Build history of the part. All positions in model axes, mm. Face numbers are marked on the shaded views. A direction names the side the tool comes from. Round coordinates to 2 decimals unless told otherwise and drop trailing zeros. Write each loop counter-clockwise with the first axis right and the second up, starting at its lowest first coordinate (ties: lowest second). Pieces come first, ordered by that corner, then holes. Notation, with made-up numbers: M -22.75,-38 L -14.75,-38 A28 ccw -14.75,-4 Z; hole C -24.75,28.25 d2. An arc over 180 degrees is marked long. Write item = value, one per line.
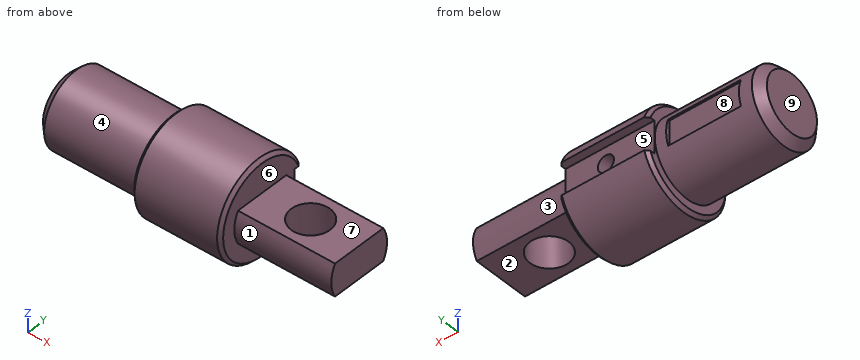
from build123d import *

# Parameters (mm, degrees)
SKETCH_2_W                  = 45
SKETCH_2_H                  = 2.5
CUT_EXTRUDE_1_DEPTH         = 8
SKETCH_4_W                  = 20
SKETCH_4_H                  = 6.715728753
CUT_EXTRUDE_2_DEPTH         = 123.576506721
HOLE_WIZARD_10_0_10_1_D     = 10
HOLE_WIZARD_10_0_10_1_DEPTH = 35
HOLE_WIZARD_10_0_10_1_TIP   = 3.004303095
CUT_EXTRUDE_START           = -60
CUT_EXTRUDE_3_DEPTH         = 245.932420089
HOLE_WIZARD_24_0_24_1_D     = 24
CHAMFER_1_SIZE              = 5
CHAMFER_2_SIZE              = 2


with BuildPart() as part:
    # Эскиз1 → Повернуть1 (revolve)
    with BuildSketch(Plane.XY, mode=Mode.PRIVATE) as revolve_1_sk:
        Polygon((0, 0), (0, 23), (65, 23), (65, 30), (120, 30), (120, 20), (180, 20), (180, 0), align=None)
    revolve(revolve_1_sk.sketch.rotate(Axis((0, 0, 0), (-1, 0, 0)), 90), axis=Axis((0, 0, 0), (-1, 0, 0)))

    # Эскиз2 → Вырез-Вытянуть1 (cut, symmetric)
    with BuildSketch(Plane.XY):
        with Locations((35.5, 21.75)):
            Rectangle(SKETCH_2_W, SKETCH_2_H)
    extrude(amount=CUT_EXTRUDE_1_DEPTH, both=True, mode=Mode.SUBTRACT)

    # Эскиз4 → Вырез-Вытянуть2 (cut, through all)
    with BuildSketch(Plane.ZY.offset(-65)):
        with Locations((0, 26.642135624)):
            Rectangle(SKETCH_4_W, SKETCH_4_H)
    extrude(amount=-CUT_EXTRUDE_2_DEPTH, mode=Mode.SUBTRACT)

    # Диаметр отверстия Ø10.0 (10)1
    with Locations(Plane(origin=(0, 23.284271247, 0), x_dir=(1, 0, 0), z_dir=(0, 1, 0))):
        with Locations((95, 0)):
            Hole(HOLE_WIZARD_10_0_10_1_D / 2, depth=HOLE_WIZARD_10_0_10_1_DEPTH)
            with Locations((0, 0, -(HOLE_WIZARD_10_0_10_1_DEPTH + HOLE_WIZARD_10_0_10_1_TIP / 2))):  # 118° drill point
                Cone(0, HOLE_WIZARD_10_0_10_1_D / 2, HOLE_WIZARD_10_0_10_1_TIP, mode=Mode.SUBTRACT)

    # Эскиз7 → Вырез-Вытянуть3 (cut)
    with BuildSketch(Plane(origin=(180, 0, 0), x_dir=(0, 0, -1), z_dir=(1, 0, 0)).offset(CUT_EXTRUDE_START)):
        Polygon((-10, 151.24355653), (-10, 17.320508076), (-10, -17.320508076), (-10, -151.24355653), (-277.846096908, -151.24355653), (-277.846096908, 151.24355653), align=None)
    cut_extrude_3 = extrude(amount=CUT_EXTRUDE_3_DEPTH, mode=Mode.SUBTRACT)

    # Зеркальное отражение1: Вырез-Вытянуть3 across plane
    add(cut_extrude_3.mirror(Plane.XY), mode=Mode.SUBTRACT)

    # Диаметр отверстия Ø24.0 (24)1 (through all)
    with Locations(Plane.XY.offset(10)):
        with Locations((150, 0)):
            Hole(HOLE_WIZARD_24_0_24_1_D / 2)

    # Фаска1
    chamfer_1_edges = [part.edges().sort_by_distance(p)[0] for p in [
        (0, 0, 23),
    ]]
    chamfer(chamfer_1_edges, length=CHAMFER_1_SIZE)

    # Фаска2
    chamfer_2_edges = [part.edges().sort_by_distance(p)[0] for p in [
        (120, -30, 0),
        (65, -30, 0),
    ]]
    chamfer(chamfer_2_edges, length=CHAMFER_2_SIZE)


solid = part.part
1. Band-saw the part on C-C (x = 63). List the corners of the cut face in (y, z), plus the area to 3 significant figures.
Responses:
outline = C 0,0 d46
area = 1,660 mm²
2. Tool access for the marked faces 1, 2, 3, 4 and 5: list every direction of +Z, -Z, +X, -X, +Y, -Y with a clear straight run to the whole face (end or side of a thin tool).
Responses:
face_1 = +X, -Y
face_2 = -Z, +X, +Y, -Y
face_3 = +X, +Y
face_4 = -X
face_5 = +X, -X, +Y
3. Band-saw the part on B-B (x = 150). List the corners of the cut face in (y, z).
Responses:
outline = M -17.32,-10 L -12,-10 L -12,10 L -17.32,10 A20 ccw Z; M 12,-10 L 17.32,-10 A20 ccw 17.32,10 L 12,10 Z
4. Flat gauge pins, fed straight in: pin 1 (17.5 mm diameter, centred on x = 138, y = -2.5, fed in from +Z); pin 2 (2 mm diameter, centred on x = 121.5, y = 12.5, fed in from -Z); pin 3 (12 mm diameter, centred on x = 136.5, z = 3.5, fed in from -Y). Where does each tip first touch, or does it go through?
Responses:
pin_1 = 10
pin_2 = -10
pin_3 = -20
5. Probe probe 1 along Z at (x, y) = (95, 11); probe 2 along Z at (x, y) = (159, 8.5); probe 3 along Z at (x, y) = (95, -2). List the from-to ranges inside material, lowest first.
Responses:
probe_1 = -27.91 to -5, 5 to 27.91
probe_2 = -10 to 10
probe_3 = -29.93 to -5, 5 to 29.93
6. Band-saw the part on A-A (y = 0). List the corners of the cut face in (x, z), plus the area to 3 significant figures.
Responses:
outline = M 0,-18 L 5,-23 L 65,-23 L 65,-28 L 67,-30 L 118,-30 L 120,-28 L 120,-10 L 138,-10 L 138,10 L 120,10 L 120,28 L 118,30 L 67,30 L 65,28 L 65,23 L 5,23 L 0,18 Z; M 162,-10 L 180,-10 L 180,10 L 162,10 Z; hole C 95,0 d10
area = 6,900 mm²
7. Band-saw the part on D-D (x = 103.5). List the corners of the cut face in (y, z).
Responses:
outline = M 23.28,-10 L 23.28,10 L 28.28,10 A30 ccw long 28.28,-10 Z
8. Mould opens along X. For the marked faces 6, 7, 8 and 9 say: pulls with the +X half, pulls with the -X half, needs draft (parallel to the pull), parting line crosses it, or undercut.
Responses:
face_6 = pulls with the +X half
face_7 = needs draft
face_8 = undercut
face_9 = pulls with the -X half
